Read the model definition and answer for the solid it produces. Units are mm, in the model's axes. Face numbers are marked on the shaded views. A direction names the side the tool comes from. Coordinates: 2 decimals unless noted, no trailing zeros. One line per item, written item: value. Start each with the question number.
```python
from build123d import *

# Parameters (mm, degrees)
F2_R     = 5.05
F3_DEPTH = 1
F4_R     = 4
F5_DEPTH = 3.4


with BuildPart() as f1:
    # F0 (on Front) → F1 (revolve)
    with BuildSketch(Plane.XZ):
        with BuildLine():
            Line((-7.9909514666, 2.4), (-9.5, 2.4))
            Line((-9.5, 2.4), (-9.5, 0.4530665231))
            Line((-9.5, 0.4530665231), (-9.0727129846, 0))
            Line((-9.0727129846, 0), (0, 0))
            Line((0, 0), (0, 1.4471871546))
            add(Edge.make_bspline(
                [(-7.9909514666, 2.4), (-7.9909515723, 1.617711094), (-2.9710125266, 1.4720783209), (-1.7912473995, 1.4308859827), (0, 1.4471871546)],
                knots=[0, 0, 0, 0, 0.5112998469, 1, 1, 1, 1], degree=3))
        make_face()
    revolve(axis=Axis((0, 0, 1.4471871546), (0, 0, -1)))

    # F2 (on face) → F3 (join)
    with BuildSketch(Plane(origin=(0, 0, 0), x_dir=(1, 0, 0), z_dir=(0, 0, -1))):
        Circle(F2_R)
    extrude(amount=F3_DEPTH)

    # F4 (on face) → F5 (join)
    with BuildSketch(Plane(origin=(0, 0, -1), x_dir=(1, 0, 0), z_dir=(0, 0, -1))):
        Circle(F4_R)
    extrude(amount=F5_DEPTH)


solid = f1.part
```
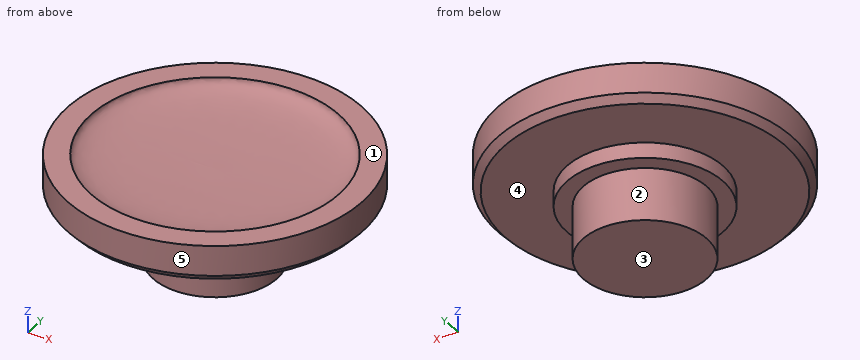
1) For a pull along Z with two mould halves and no side action, classify the marked faces 1, 2 and 3 as released by +Z, released by -Z, zero draft, split by the parting line, or undercut.
2) Consider line 1 along Z through (x, y) = (7.5, 4.75); line 2 along Y through (x, z) = (-7.25, 2.25); line 3 along Y through (x, z) = (-0.5, 1). Determine where each line is inside the solid, lowest interval first.
3) Flat-ended cylindrical pins translate along their axes: pin 1 (2 mm diameter, centred on y = 3.5, z = 0, fed in from +X); pin 2 (1.5 mm diameter, centred on x = -4.5, z = 0, fed in from +Y). Find the tip coordinate at first contact, or state that the pin passes through.
4) A tool of negligible diameter and unlimited length cuts with its end or side. For the marked faces 4 and 5, from which of +Z, -Z, +X, -X, +Y, -Y can it reach the whole face along a straight path? Write none if from no direction.
Results found:
1. face 1: released by +Z
1. face 2: zero draft
1. face 3: released by -Z
2. line 1: z = 0 to 2.4
2. line 2: y = -6.14 to -3.28, 3.28 to 6.14
2. line 3: y = -9.49 to 9.49
3. pin 1: stops at x = 9.13
3. pin 2: stops at y = 8.66
4. face 4: -Z
4. face 5: +Z, -Z
